```python
from build123d import *

# Parameters (mm, degrees)
ESQUISSE1_W             = 78.22
ESQUISSE1_H             = 78.22
BOSS_EXTRU_1_DEPTH      = 22
COQUE1_T                = -8
ESQUISSE2_R             = 2
ENL_V_MAT_EXTRU_1_DEPTH = 14
ESQUISSE3_R             = 3.5
BOSS_EXTRU_2_DEPTH      = 5
ESQUISSE3_4_R           = 1
ENL_V_MAT_EXTRU_3_DEPTH = 5
ESQUISSE6_R             = 2.5
ENL_V_MAT_EXTRU_4_DEPTH = 12


with BuildPart() as part:
    # Esquisse1 → Boss.-Extru.1 (new body)
    with BuildSketch(Plane.XY):
        Rectangle(ESQUISSE1_W, ESQUISSE1_H)
    extrude(amount=BOSS_EXTRU_1_DEPTH)

    # Coque1
    coque1_openings = [part.faces().sort_by_distance(p)[0] for p in [
        (0, 0, 22),
    ]]
    offset(amount=COQUE1_T, openings=coque1_openings, kind=Kind.INTERSECTION)

    # Esquisse2 → Enl_v. mat.-Extru.1 (cut)
    with BuildSketch(Plane.XY.offset(22)):
        with Locations((-35.11, 35.11)):
            Circle(ESQUISSE2_R)
        with Locations((35.11, -35.11)):
            Circle(ESQUISSE2_R)
        with Locations((35.11, 35.11)):
            Circle(ESQUISSE2_R)
        with Locations((-35.11, -35.11)):
            Circle(ESQUISSE2_R)
    extrude(amount=-ENL_V_MAT_EXTRU_1_DEPTH, mode=Mode.SUBTRACT)

    # Esquisse3 → Boss.-Extru.2 (add)
    with BuildSketch(Plane.XY.offset(8)):
        with Locations((-21.65, 26.75)):
            Circle(ESQUISSE3_R)
        with Locations((-21.65, -26.75)):
            Circle(ESQUISSE3_R)
        with Locations((21.65, -26.75)):
            Circle(ESQUISSE3_R)
        with Locations((21.65, 26.75)):
            Circle(ESQUISSE3_R)
    extrude(amount=BOSS_EXTRU_2_DEPTH)

    # Esquisse3_4 → Enl_v. mat.-Extru.3 (cut)
    with BuildSketch(Plane.XY.offset(8)):
        with Locations((-21.65, 26.75)):
            Circle(ESQUISSE3_4_R)
        with Locations((-21.65, -26.75)):
            Circle(ESQUISSE3_4_R)
        with Locations((21.65, -26.75)):
            Circle(ESQUISSE3_4_R)
        with Locations((21.65, 26.75)):
            Circle(ESQUISSE3_4_R)
    extrude(amount=ENL_V_MAT_EXTRU_3_DEPTH, mode=Mode.SUBTRACT)

    # Esquisse6 → Enl_v. mat.-Extru.4 (cut)
    with BuildSketch(Plane.ZY.offset(39.11)):
        with Locations((12, -0.040287358)):
            Circle(ESQUISSE6_R)
    extrude(amount=-ENL_V_MAT_EXTRU_4_DEPTH, mode=Mode.SUBTRACT)


solid = part.part
```
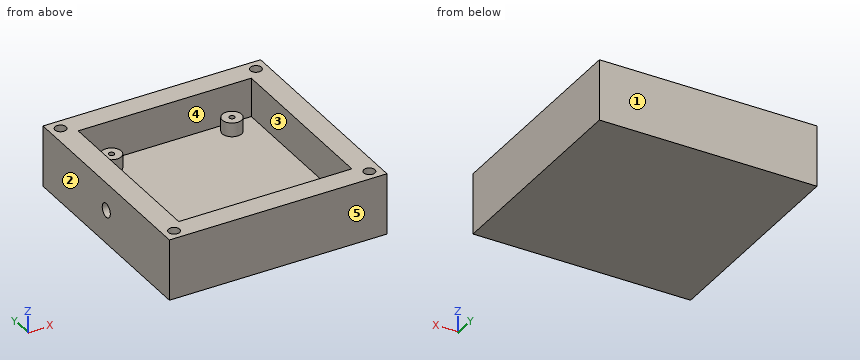
Check sheet for the modelled part. Datum: model origin and axes. Units: mm. Face numbers are marked on the shaded views. A direction names the side the tool comes from. Round coordinates to 2 decimals unless told otherwise and drop trailing zeros. Loops run counter-clockwise (first coordinate to the right, second up) from the corner with the lowest first, then second, coordinate; pieces in that order, holes last. Notation, with made-up numbers: (54.5, -20) -> (106.5, -20) arc R13 cw to (106.5, -5) -> close; hole circle Ø6 at (80, 5.5). An arc over 180 degrees is marked (long way). Write item = value, one per line. Start each with the question number.
1) Sectioned sample at C-C, the plane z = 16.25. Record the cut outline in (x, y).
2) Thickness scan on probe 1 along Y at (x, z) = (21.65, 9); probe 2 along Y at (x, z) = (-35.11, 18.5); probe 3 along X at (y, z) = (14.5, 14.5). Record the ranges inside material, lowest first.
3) Set-up check for the marked faces 4 and 5: record each of +Z, -Z, +X, -X, +Y, -Y from which the full face is reachable in a straight line by a thin tool's end or side.
4) Sectioned sample at A-A, the plane y = 35.11. Record the cut outline in (x, z), plus the area to 3 significant figures.
5) Release check for a two-part mould opening along Y. For the marked faces 1, 2 and 3 record: released by +Y, released by -Y, zero draft, split by the parting line, or undercut.
6) Sectioned sample at B-B, the plane x = -21.65. Record the cut outline in (y, z), plus the area to 3 significant figures.
7) Sectioned sample at D-D, the plane y = 4. Record the cut outline in (x, z).
8) Gauge pin test, flat ends, axial feed: pin 1 Ø3 at (x, y) = (-34, -35) entering from +Z; pin 2 Ø2 at (x, y) = (-6, -20.5) entering from +Z; pin 3 Ø3 at (x, y) = (-21.65, 26.75) entering from +Z. Record the tip position at first contact, or that the pin passes through.
Results are:
q1.outline = (-39.11, -39.11) -> (39.11, -39.11) -> (39.11, 39.11) -> (-39.11, 39.11) -> close; hole circle Ø4 at (-35.11, -35.11); hole circle Ø4 at (-35.11, 35.11); hole (-31.11, -31.11) -> (31.11, -31.11) -> (31.11, 31.11) -> (-31.11, 31.11) -> close; hole circle Ø4 at (35.11, -35.11); hole circle Ø4 at (35.11, 35.11)
q2.probe_1 = -39.11 to -31.11, -30.25 to -27.75, -25.75 to -23.25, 23.25 to 25.75, 27.75 to 30.25, 31.11 to 39.11
q2.probe_2 = -39.11 to -37.11, -33.11 to 33.11, 37.11 to 39.11
q2.probe_3 = -39.11 to -31.11, 31.11 to 39.11
q3.face_4 = +Z
q3.face_5 = +Z, -Z, +X, -X, -Y
q4.outline = (-39.11, 0) -> (39.11, 0) -> (39.11, 22) -> (37.11, 22) -> (37.11, 8) -> (33.11, 8) -> (33.11, 22) -> (-33.11, 22) -> (-33.11, 8) -> (-37.11, 8) -> (-37.11, 22) -> (-39.11, 22) -> close
q4.area = 1,610 mm^2
q5.face_1 = released by +Y
q5.face_2 = zero draft
q5.face_3 = undercut
q6.outline = (-39.11, 0) -> (39.11, 0) -> (39.11, 22) -> (31.11, 22) -> (31.11, 8) -> (30.25, 8) -> (30.25, 13) -> (27.75, 13) -> (27.75, 8) -> (25.75, 8) -> (25.75, 13) -> (23.25, 13) -> (23.25, 8) -> (-23.25, 8) -> (-23.25, 13) -> (-25.75, 13) -> (-25.75, 8) -> (-27.75, 8) -> (-27.75, 13) -> (-30.25, 13) -> (-30.25, 8) -> (-31.11, 8) -> (-31.11, 22) -> (-39.11, 22) -> close
q6.area = 900 mm^2
q7.outline = (-39.11, 0) -> (39.11, 0) -> (39.11, 22) -> (31.11, 22) -> (31.11, 8) -> (-31.11, 8) -> (-31.11, 22) -> (-39.11, 22) -> close
q8.pin_1 = 22
q8.pin_2 = 8
q8.pin_3 = 13
